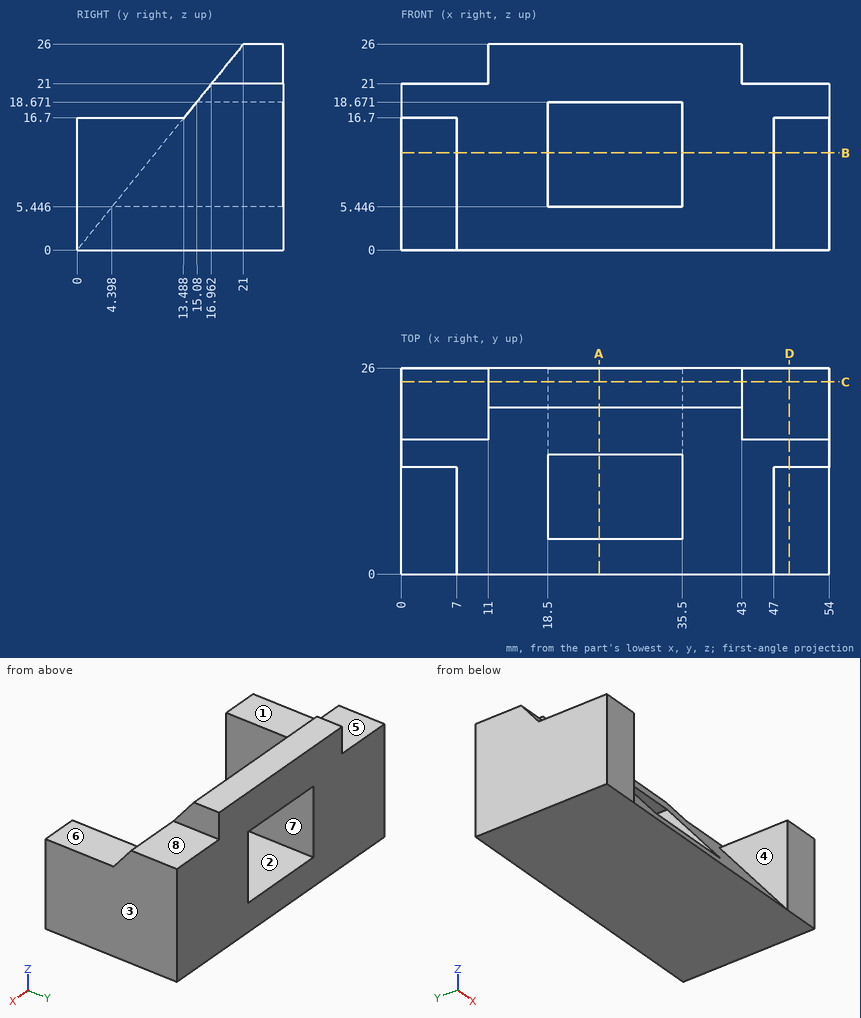
Verification items for this drawing (mm, ordinates from the low corner). A direction names the side the tool comes from. Coordinates: 2 decimals unless noted, no trailing zeros. Order: outer loops, then holes, each group sorted by start corner. A loop starts at its lowest first (then second) coordinate and runs counter-clockwise, first axis right, second up. Notation, with made-up numbers: (26.25, 85) -> (31.25, 85) arc R28 ccw to (31.25, 124) -> close; hole circle Ø9 at (-35.5, 10.5). An arc over 180 degrees is marked (long way). Put each result on its own line as item: value. Start each with the question number.
1. Go/stop test with flat-tipped pins: pin 1 Ø6 at (x, y) = (19, 7) entering from +Z; pin 2 Ø10 at (x, y) = (5.5, 11.5) entering from +Z; pin 3 Ø7 at (x, y) = (49.5, 21.5) entering from +Z. Record where each tip stops, or that it passes through.
2. Mould release check, pull along X, two halves, no side actions. Record for the marked faces 1, 2 and 3: released by +X, released by -X, zero draft, split by the parting line, or undercut.
3. Cross-section at C-C, the plane y = 24.25. Record the boundary of the cut face in (x, z) (1 decimal), then the cut area to 3 significant figures.
4. Cross-section at B-B, the plane z = 12.25. Record the boundary of the cut face in (x, y) (1 decimal).
5. Cross-section at A-A, the plane x = 25. Record the boundary of the cut face in (y, z) (1 decimal), then the cut area to 3 significant figures.
6. Access from +Z, -Z, +X, -X, +Y, -Y to the whole of each face (thin tool, end or side, straight path). Record for the marked faces 4, 5, 6, 7 and 8.
7. Material ranges on L1, parallel to X at y = 12.5, z = 10.5; L2, parallel to X at y = 4.75, z = 8.75; L3, parallel to Z at x = 23, y = 10.75 (1 decimal), recorded low to high. Write a range as [from, to].
8. Cross-section at D-D, the plane x = 49. Record the boundary of the cut face in (y, z).
Computed:
1. pin 1: z = 12.33
1. pin 2: z = 20.43
1. pin 3: z = 21
2. face 1: zero draft
2. face 2: undercut
2. face 3: released by +X
3. outline: (0, 0) -> (54, 0) -> (54, 21) -> (43, 21) -> (43, 26) -> (11, 26) -> (11, 21) -> (0, 21) -> close; hole (18.5, 5.4) -> (35.5, 5.4) -> (35.5, 18.7) -> (18.5, 18.7) -> close
3. area: 1,070 mm2
4. outline: (0, 0) -> (7, 0) -> (7, 9.9) -> (18.5, 9.9) -> (18.5, 26) -> (0, 26) -> close; (35.5, 9.9) -> (47, 9.9) -> (47, 0) -> (54, 0) -> (54, 26) -> (35.5, 26) -> close
5. outline: (0, 0) -> (26, 0) -> (26, 5.4) -> (4.4, 5.4) -> close; (15.1, 18.7) -> (26, 18.7) -> (26, 26) -> (21, 26) -> close
5. area: 188 mm2
6. face 4: +Z, -Y
6. face 5: +Z, -X, +Y, -Y
6. face 6: +Z, +X, -X, -Y
6. face 7: +Y, -Y
6. face 8: +Z, +X, +Y, -Y
7. L1: [0, 18.5], [35.5, 54]
7. L2: [0, 7], [47, 54]
7. L3: [0, 5.4]
8. outline: (0, 0) -> (26, 0) -> (26, 21) -> (16.96, 21) -> (13.49, 16.7) -> (0, 16.7) -> close
